```python
from build123d import *

# Parameters (mm, degrees)
F1_DEPTH = 15.748
F2_W     = 72.411287576
F2_H     = 40.2284925804
F3_DEPTH = 0.508


with BuildPart() as f1:
    # F0 (on Front) → F1 (new body, symmetric)
    with BuildSketch(Plane.XZ):
        Polygon((-33.3747491241, 14.154468663), (-59.001788497, 14.154468663), (-59.001788497, -56.1708956957), (64.6635815501, -56.1708956957), (64.6635815501, 14.154468663), (39.0365384519, 14.154468663), (39.0365384519, -26.0740239173), (-33.3747491241, -26.0740239173), align=None)
    extrude(amount=F1_DEPTH, both=True)

    # F2 (on face) → F3 (join)
    with BuildSketch(Plane(origin=(0, 15.748, 0), x_dir=(-1, 0, 0), z_dir=(0, 1, 0))):
        with Locations((-2.8308946639, -5.9597776271)):
            Rectangle(F2_W, F2_H)
    extrude(amount=-F3_DEPTH)


solid = f1.part
```
Geometry check sheet. Reference: the model listing, model coordinates, mm. A direction names the side the tool comes from. Round coordinates to 2 decimals unless told otherwise and drop trailing zeros. Loops run counter-clockwise (first coordinate to the right, second up) from the corner with the lowest first, then second, coordinate; pieces in that order, holes last. Notation, with made-up numbers: (-27, 41.5) -> (-9, 41.5) arc R20 cw to (-9, 79.5) -> close; hole circle Ø7 at (59.5, 25). An arc over 180 degrees is marked (long way). Use a Markdown table: item, result.
(1) Go/stop test with a flat-tipped pin: P1, Ø10, axis at x = 6, z = -16.5, coming from the -Y side. Record where the tip stops, or that it passes through.
Calculated:
| item | result |
|---|---|
| P1 | y = 15.24 |
(2) Sectioned sample at A-A (y = -10). Enter the section's corners in (x, z).
Calculated:
| item | result |
|---|---|
| outline | (-59, -56.17) -> (64.66, -56.17) -> (64.66, 14.15) -> (39.04, 14.15) -> (39.04, -26.07) -> (-33.37, -26.07) -> (-33.37, 14.15) -> (-59, 14.15) -> close |
(3) Sectioned sample at C-C (x = -32). Enter the section's corners in (y, z).
Calculated:
| item | result |
|---|---|
| outline | (-15.75, -56.17) -> (15.75, -56.17) -> (15.75, 14.15) -> (15.24, 14.15) -> (15.24, -26.07) -> (-15.75, -26.07) -> close |
(4) Sectioned sample at B-B (z = -1). Enter the section's corners in (x, y).
Calculated:
| item | result |
|---|---|
| outline | (-59, -15.75) -> (-33.37, -15.75) -> (-33.37, 15.24) -> (39.04, 15.24) -> (39.04, -15.75) -> (64.66, -15.75) -> (64.66, 15.75) -> (-59, 15.75) -> close |
(5) Set-up check for faces 1 (the flat face through (39.037, 0, -6)), 2 (the flat face through (2, -15.748, -28)): record each of +Z, -Z, +X, -X, +Y, -Y from which the full face is reachable in a straight line by a thin tool's end or side.
Calculated:
| item | result |
|---|---|
| face 1 | +Z, -Y |
| face 2 | +Z, -Z, +X, -X, -Y |
(6) Mould release check, pull along X, two halves, no side actions. Record for faces 3 (the flat face through (45, 0, 14.154)), 4 (the flat face through (3, 0, -26.074)), 5 (the flat face through (64.664, 0, -22)): released by +X, released by -X, zero draft, split by the parting line, or undercut.
Calculated:
| item | result |
|---|---|
| face 3 | zero draft |
| face 4 | undercut |
| face 5 | released by +X |
(7) Scan lines: probe 1 along X at (y, z) = (1, -15); probe 2 along Y at (x, z) = (-27.5, -24); probe 3 along Z at (x, y) = (14, 14.5). Record each from-to range of solid material in increasing order.
Calculated:
| item | result |
|---|---|
| probe 1 | -59 to -33.37, 39.04 to 64.66 |
| probe 2 | 15.24 to 15.75 |
| probe 3 | -56.17 to -26.07 |
